Source: CAD feature listing. Evaluate the final solid. Frame: model axes, mm. A direction names the side the tool comes from. Give positions to 0.01 mm unless a question says otherwise; leave off trailing zeros. Loops run counter-clockwise (first coordinate to the right, second up) from the corner with the lowest first, then second, coordinate; pieces in that order, holes last. Notation, with made-up numbers: M 1,72.5 L 29,72.5 A34 ccw 29,103.5 Z; hole C 27,14.25 d11. An arc over 180 degrees is marked long. Put each result on its own line as item: value.
from build123d import *

# Parameters (mm, degrees)
SKETCH1_R           = 1.4
BOSS_EXTRUDE1_DEPTH = 3


with BuildPart() as part:
    # Sketch1 → Boss-Extrude1 (new body)
    with BuildSketch(Plane(origin=(0, 0, 0), x_dir=(1, 0, 0), z_dir=(0, 1, 0))):
        with BuildLine():
            Line((25.742531042, 14.690082128), (11.491487674, 28.941125497))
            ThreePointArc((11.491487674, 28.941125497), (9.869370929, 30.024989254), (7.955953768, 30.405591591))
            Line((7.955953768, 30.405591591), (0.784380892, 30.405591591))
            ThreePointArc((0.784380892, 30.405591591), (-1.129036269, 30.024989254), (-2.751153014, 28.941125497))
            Line((-2.751153014, 28.941125497), (-24.570958167, 7.121320344))
            ThreePointArc((-24.570958167, 7.121320344), (-25.654821924, 5.499203599), (-26.035424261, 3.585786438))
            Line((-26.035424261, 3.585786438), (-26.035424261, -3.585786438))
            ThreePointArc((-26.035424261, -3.585786438), (-25.654821924, -5.499203599), (-24.570958167, -7.121320344))
            Line((-24.570958167, -7.121320344), (-2.751153014, -28.941125497))
            ThreePointArc((-2.751153014, -28.941125497), (-1.129036269, -30.024989254), (0.784380892, -30.405591591))
            Line((0.784380892, -30.405591591), (7.955953768, -30.405591591))
            ThreePointArc((7.955953768, -30.405591591), (9.869370929, -30.024989254), (11.491487674, -28.941125497))
            Line((11.491487674, -28.941125497), (25.742531042, -14.690082128))
            Line((25.742531042, -14.690082128), (25.742531042, -13.305049063))
            ThreePointArc((25.742531042, -13.305049063), (23.11272458, -10.777668219), (21.090366856, -7.742276119))
            Line((21.090366856, -7.742276119), (19.392389552, -7.742276119))
            ThreePointArc((19.392389552, -7.742276119), (-12.529702293, -0.066383131), (19.331103203, 7.860050751))
            Line((19.331103203, 7.860050751), (21.039064127, 7.860050751))
            ThreePointArc((21.039064127, 7.860050751), (23.086785029, 10.90224193), (25.742531042, 13.431095658))
            Line((25.742531042, 13.431095658), (25.742531042, 14.690082128))
        make_face()
        with Locations((12.501895314, -22.273863607)):
            Circle(SKETCH1_R, mode=Mode.SUBTRACT)
        with Locations((-3.761560654, -22.273863607)):
            Circle(SKETCH1_R, mode=Mode.SUBTRACT)
        with Locations((-17.903696277, -8.131727984)):
            Circle(SKETCH1_R, mode=Mode.SUBTRACT)
        with Locations((-17.903696277, 8.131727984)):
            Circle(SKETCH1_R, mode=Mode.SUBTRACT)
        with Locations((-3.761560654, 22.273863607)):
            Circle(SKETCH1_R, mode=Mode.SUBTRACT)
        with Locations((12.501895314, 22.273863607)):
            Circle(SKETCH1_R, mode=Mode.SUBTRACT)
    extrude(amount=BOSS_EXTRUDE1_DEPTH)


solid = part.part
1. Material intervals for line 1 (Z direction, x = 16, y = 0.8); line 2 (Z direction, x = -18.5, y = 1.8); line 3 (Z direction, x = 2.5, y = 2.1), sorted ascending. Write a range as from..to.
Found:
line 1: -24.43..-12.26, 12.26..24.43
line 2: -13.19..-9.4, -6.87..6.87, 9.4..13.19
line 3: -30.41..-16.8, 16.8..30.41
2. Draft query along Z for faces 3 (the cylindrical face through (23.05, 1.48, -10.86)), 4 (the flat face through (4, 1, 30.406)), 5 (the flat face through (4, 1, -30.406)). Return one class per face: pulls with the +Z half, pulls with the -Z half, needs draft (parallel to the pull), parting line crosses it, or undercut.
Found:
face 3: undercut
face 4: pulls with the +Z half
face 5: pulls with the -Z half
3. Section query C-C (x = 17). Output: boundary loops of the cut face in (y, z), plus the area to 3 significant figures.
Found:
outline: M 0,-23.43 L 3,-23.43 L 3,-11.23 L 0,-11.23 Z; M 0,11.23 L 3,11.23 L 3,23.43 L 0,23.43 Z
area: 73.2 mm^2
4. Contact query for flat-ended pins moving along their axis: P1, Ø2, axis at x = -3.76, z = -22.27, coming from the +Y side; P2, Ø1.4, axis at x = 20, y = 1.5, coming from the -Z side. Output: stop coordinate, or through.
Found:
P1: through
P2: z = -21.13
5. Access query for faces 1 (the flat face through (20, 1, 7.742)), 2 (the flat face through (18.717, 1.479, -21.716)). Directions: +Z, -Z, +X, -X, +Y, -Y. A direction counts if a zero-diameter tool reaches every point of the face in a straight line with its end or side. Return the directions, or none.
Found:
face 1: +X, +Y, -Y
face 2: -Z, +X, +Y, -Y
6. Section query A-A (x = -8.5). Output: boundary loops of the cut face in (y, z), plus the area to 3 significant figures.
Found:
outline: M 0,-23.19 L 3,-23.19 L 3,-10.95 L 0,-10.95 Z; M 0,10.95 L 3,10.95 L 3,23.19 L 0,23.19 Z
area: 73.4 mm^2
7. Section query B-B (y = 1.5). Output: boundary loops of the cut face in (x, z).
Found:
outline: M -26.04,-3.59 A5 ccw -24.57,-7.12 L -2.75,-28.94 A5 ccw 0.78,-30.41 L 7.96,-30.41 A5 ccw 11.49,-28.94 L 25.74,-14.69 L 25.74,-13.43 A16.9 cw 21.04,-7.86 L 19.33,-7.86 A16.9 cw long 19.39,7.74 L 21.09,7.74 A16.8 cw 25.74,13.31 L 25.74,14.69 L 11.49,28.94 A5 ccw 7.96,30.41 L 0.78,30.41 A5 ccw -2.75,28.94 L -24.57,7.12 A5 ccw -26.04,3.59 Z; hole C -17.9,-8.13 d2.8; hole C -17.9,8.13 d2.8; hole C -3.76,-22.27 d2.8; hole C -3.76,22.27 d2.8; hole C 12.5,-22.27 d2.8; hole C 12.5,22.27 d2.8
8. Section query D-D (z = 0). Output: boundary loops of the cut face in (x, y).
Found:
outline: M -26.04,0 L -12.53,0 L -12.53,3 L -26.04,3 Z
